Geometry check sheet. Reference: the model listing, model coordinates, mm. A direction names the side the tool comes from. Coordinates: 2 decimals unless noted, no trailing zeros. Loops run counter-clockwise (first coordinate to the right, second up) from the corner with the lowest first, then second, coordinate; pieces in that order, holes last. Notation, with made-up numbers: (-18, -31) -> (-12, -31) arc R21 ccw to (-12, -23) -> close; hole circle Ø8 at (89, 76.5). An arc over 180 degrees is marked (long way). Answer as a JSON object with one key per item and string values.
from build123d import *

# Parameters (mm, degrees)
SKETCH1_R           = 7.5311
SKETCH1_R_2         = 5.969
BOSS_EXTRUDE1_DEPTH = 0.5588
SKETCH2_W           = 1.834896806
SKETCH2_H           = 1.901806754
CUT_EXTRUDE1_DEPTH  = 1.5588
CIRPATTERN1_COUNT   = 10


with BuildPart() as part:
    # Sketch1 → Boss-Extrude1 (new body)
    with BuildSketch(Plane(origin=(0, 0, 0), x_dir=(1, 0, 0), z_dir=(0, 1, 0))):
        Circle(SKETCH1_R)
        Circle(SKETCH1_R_2, mode=Mode.SUBTRACT)
    extrude(amount=BOSS_EXTRUDE1_DEPTH)

    # Sketch2 → Cut-Extrude1 (cut, through all)
    with BuildSketch(Plane(origin=(0, 0.5588, 0), x_dir=(1, 0, 0), z_dir=(0, 1, 0))):
        with Locations((0, 5.969)):
            Rectangle(SKETCH2_W, SKETCH2_H)
    cut_extrude1 = extrude(amount=-CUT_EXTRUDE1_DEPTH, mode=Mode.SUBTRACT)

    # CirPattern1: Cut-Extrude1 ×10 about axis
    cirpattern1_axis = Axis((0, 0, 0), (0, 1, 0))
    for i in range(1, CIRPATTERN1_COUNT):
        add(cut_extrude1.rotate(cirpattern1_axis, i * 360 / CIRPATTERN1_COUNT), mode=Mode.SUBTRACT)


solid = part.part
1. Mould release check, pull along Z, two halves, no side actions. Record for faces 3 (the face through (-2, 0, -6)), 4 (the face through (-4.82, 0.28, -3.52)), 5 (the face through (-5.98, 0.28, 4.58)): released by +Z, released by -Z, zero draft, split by the parting line, or undercut.
Evaluation:
{"face 3": "zero draft", "face 4": "undercut", "face 5": "split by the parting line"}
2. Section check A-A, the plane x = 0. Record the boundary of the cut face in (y, z).
Evaluation:
{"outline": "(0, -7.53) -> (0.56, -7.53) -> (0.56, -6.92) -> (0, -6.92) -> close; (0, 6.92) -> (0.56, 6.92) -> (0.56, 7.53) -> (0, 7.53) -> close"}
3. Tool access check on faces 1 (the face through (4.82, 0.28, 3.52)), 2 (the face through (-2, 0.559, -6)). Record the directions out of +Z, -Z, +X, -X, +Y, -Y that give a thin tool (end or side, any length) a straight path to the whole face; none if there is none.
Evaluation:
{"face 1": "+Y, -Y", "face 2": "+Z, -Z, +X, -X, +Y"}
4. Thickness scan on probe 1 along Z at (x, y) = (0, 0.3); probe 2 along Z at (x, y) = (-4.5, 0.4); probe 3 along X at (y, z) = (0.1, 0). Record the ranges inside material, lowest first. Write a range as from..to.
Evaluation:
{"probe 1": "z = -7.53..-6.92, 6.92..7.53", "probe 2": "z = -6.04..-5.28, -4.63..-3.92, 3.92..4.63, 5.28..6.04", "probe 3": "x = -7.53..-5.97, 5.97..7.53"}
5. Section check B-B, the plane z = 2. Record the boundary of the cut face in (x, y).
Evaluation:
{"outline": "(-7.26, 0) -> (-6.63, 0) -> (-6.63, 0.56) -> (-7.26, 0.56) -> close; (6.63, 0) -> (7.26, 0) -> (7.26, 0.56) -> (6.63, 0.56) -> close"}
